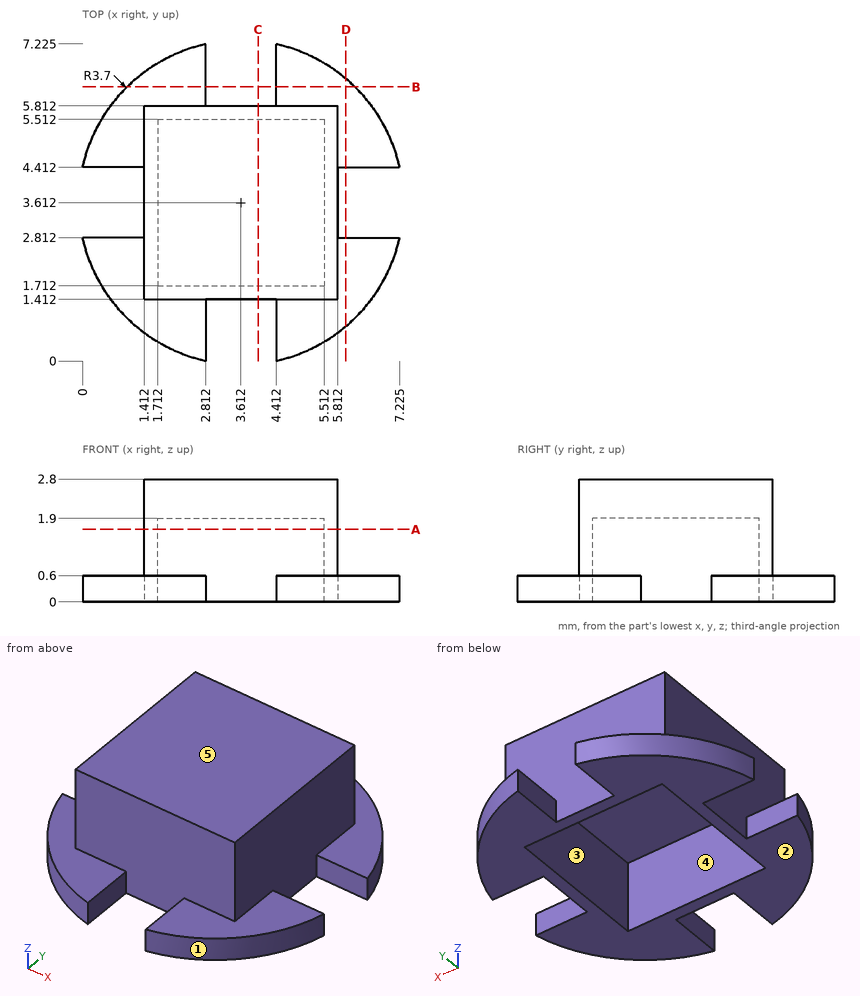
Input: dimensioned drawing with shaded views. Units: mm. Origin: part minimum x, y, z. A direction names the side the tool comes from. Coordinates: 2 decimals unless noted, no trailing zeros. Write each loop counter-clockwise with the first axis right and the second up, starting at its lowest first coordinate (ties: lowest second). Pieces come first, ordered by that corner, then holes. Notation, with made-up numbers: (38.25, -27) -> (90.25, -27) arc R8 ccw to (90.25, -19) -> close; hole circle Ø2 at (88.25, -38.5). An arc over 180 degrees is marked (long way). Return JSON: item names as keys, results as strings. Group by question number.
1) Mould query, pull axis X, two halves, no side actions, for the marked faces 1, 2 and 3. Classes: +X half, -X half, draft (parallel to the pull), parting line (faces both ways), or undercut.
2) Section query C-C, the plane x = 4. Return loops of the section in (y, z).
3) Section query D-D, the plane x = 6. Return loops of the section in (y, z) (1 decimal).
4) Ray query, line 1 along Y through (x, z) = (4.5, 1); line 2 along Z through (x, y) = (2.75, 6.5). Return the intervals inside material, ascending.
5) Contact query for flat-ended pins moving along their axis: P1, Ø1.5, axis at y = 3.5, z = 1.5, coming from the +X side; P2, Ø0.5, axis at y = 0.5, z = 0.5, coming from the -X side; P3, Ø1.4, axis at x = 4, z = 1.5, coming from the +Y side. Output: stop coordinate, or through.
6) Section query A-A, the plane z = 1.65. Return loops of the section in (x, y).
7) Section query B-B, the plane y = 6.25. Return loops of the section in (x, z).
8) Set-up query: the marked faces 4 and 5. Return all of +Z, -Z, +X, -X, +Y, -Y with unobstructed straight access to the full face (end or side cutting, diameter ignored); none if empty.
From the geometry:
{
 "1": {"face 1": "+X half", "face 2": "draft", "face 3": "undercut"},
 "2": {"outline": "(1.41, 0) -> (1.71, 0) -> (1.71, 1.9) -> (5.51, 1.9) -> (5.51, 0) -> (5.81, 0) -> (5.81, 2.8) -> (1.41, 2.8) -> close"},
 "3": {"outline": "(0.8, 0) -> (2.8, 0) -> (2.8, 0.6) -> (0.8, 0.6) -> close; (4.4, 0) -> (6.4, 0) -> (6.4, 0.6) -> (4.4, 0.6) -> close"},
 "4": {"line 1": "1.41 to 1.71, 5.51 to 5.81", "line 2": "0 to 0.6"},
 "5": {"P1": "x = 5.81", "P2": "x = 1.27", "P3": "y = 5.81"},
 "6": {"outline": "(1.41, 1.41) -> (5.81, 1.41) -> (5.81, 5.81) -> (1.41, 5.81) -> close; hole (1.71, 1.71) -> (5.51, 1.71) -> (5.51, 5.51) -> (1.71, 5.51) -> close"},
 "7": {"outline": "(1.02, 0) -> (2.81, 0) -> (2.81, 0.6) -> (1.02, 0.6) -> close; (4.41, 0) -> (6.21, 0) -> (6.21, 0.6) -> (4.41, 0.6) -> close"},
 "8": {"face 4": "-Z", "face 5": "+Z, +X, -X, +Y, -Y"}
}
